Print and shaded views of the part. All mm, measured from the part's lowest x, y and z. Give positions to 0.01 mm unless a question says otherwise; leave off trailing zeros. Loops run counter-clockwise (first coordinate to the right, second up) from the corner with the lowest first, then second, coordinate; pieces in that order, holes last. Notation, with made-up numbers: (25.5, 66.5) - (34.5, 66.5) arc R33 cw to (34.5, 95.5) - close; hole circle Ø4 at (-38.5, 58.5). An arc over 180 degrees is marked (long way). Return JSON: item names as keys, results as strings.
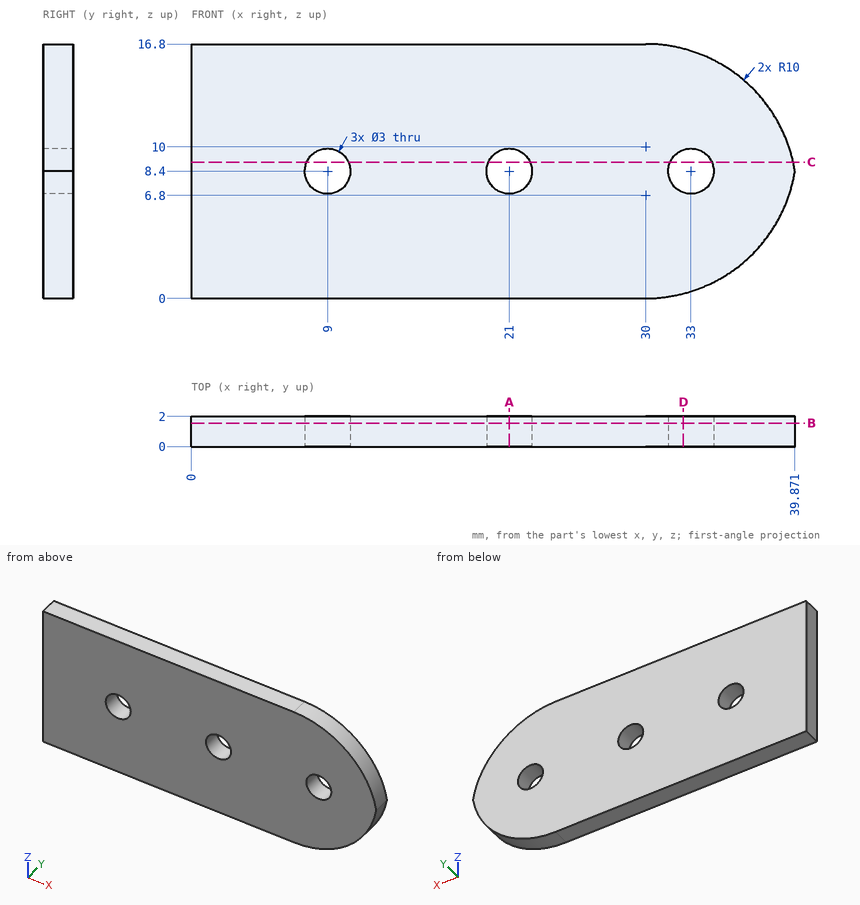
1. Cut at B-B, the plane y = 1.55. Write the cut outline in (x, z), plus the area to 3 significant figures.
Values follow:
{"outline": "(0, 0) - (30, 0) arc R10 ccw to (39.87, 8.4) arc R10 ccw to (30, 16.8) - (0, 16.8) - close; hole circle Ø3 at (9, 8.4); hole circle Ø3 at (21, 8.4); hole circle Ø3 at (33, 8.4)", "area": "608 mm²"}
2. Drill centre lines: probe 1 along Z at (x, y) = (10, 0.75); probe 2 along X at (y, z) = (0.5, 13); probe 3 along Z at (x, y) = (36, 0.75). Where is each one in solid material? Low to high.
Values follow:
{"probe 1": "z = 0 to 7.28, 9.52 to 16.8", "probe 2": "x = 0 to 37.85", "probe 3": "z = 2 to 14.8"}
3. Cut at A-A, the plane x = 21. Write the cut outline in (y, z).
Values follow:
{"outline": "(0, 0) - (2, 0) - (2, 6.9) - (0, 6.9) - close; (0, 9.9) - (2, 9.9) - (2, 16.8) - (0, 16.8) - close"}
4. Drop a flat-ended pin along its axis: P1, Ø5, axis at x = 21, z = 8.4, coming from the -Y side. Give the stop position or say it passes through.
Values follow:
{"P1": "stops at y = 0"}
5. Cut at D-D, the plane x = 32.5. Write the cut outline in (y, z).
Values follow:
{"outline": "(0, 0.32) - (2, 0.32) - (2, 6.99) - (0, 6.99) - close; (0, 9.81) - (2, 9.81) - (2, 16.48) - (0, 16.48) - close"}
6. Cut at C-C, the plane z = 9. Write the cut outline in (x, y) (1 decimal), plus the area to 3 significant figures.
Values follow:
{"outline": "(0, 0) - (7.6, 0) - (7.6, 2) - (0, 2) - close; (10.4, 0) - (19.6, 0) - (19.6, 2) - (10.4, 2) - close; (22.4, 0) - (31.6, 0) - (31.6, 2) - (22.4, 2) - close; (34.4, 0) - (39.8, 0) - (39.8, 2) - (34.4, 2) - close", "area": "63.0 mm²"}
